Work out the finished part from the listing and answer in its coordinate system (mm). Face numbers are marked on the shaded views. A direction names the side the tool comes from. Coordinates: 2 decimals unless noted, no trailing zeros. Order: outer loops, then holes, each group sorted by start corner. A loop starts at its lowest first (then second) coordinate and runs counter-clockwise, first axis right, second up. Notation, with made-up numbers: M 8.5,10.5 L 35.5,10.5 A10 cw 35.5,27.5 Z; hole C 14,45.5 d4. An arc over 180 degrees is marked long. Use a Markdown table: item, result.
from build123d import *

# Parameters (mm, degrees)
SKETCH1_R           = 15
BOSS_EXTRUDE1_DEPTH = 10
SKETCH2_R           = 7
BOSS_EXTRUDE2_DEPTH = 98
SKETCH4_R           = 15
BOSS_EXTRUDE3_DEPTH = 10


with BuildPart() as part:
    # Sketch1 → Boss-Extrude1 (new body)
    with BuildSketch(Plane(origin=(0, 0, 0), x_dir=(1, 0, 0), z_dir=(0, 1, 0))):
        Circle(SKETCH1_R)
    extrude(amount=-BOSS_EXTRUDE1_DEPTH)

    # Sketch2 → Boss-Extrude2 (add)
    with BuildSketch(Plane.XZ.offset(10)):
        Circle(SKETCH2_R)
    extrude(amount=BOSS_EXTRUDE2_DEPTH)

    # Sketch4 → Boss-Extrude3 (add)
    with BuildSketch(Plane.XZ.offset(108)):
        Circle(SKETCH4_R)
    extrude(amount=-BOSS_EXTRUDE3_DEPTH)


solid = part.part
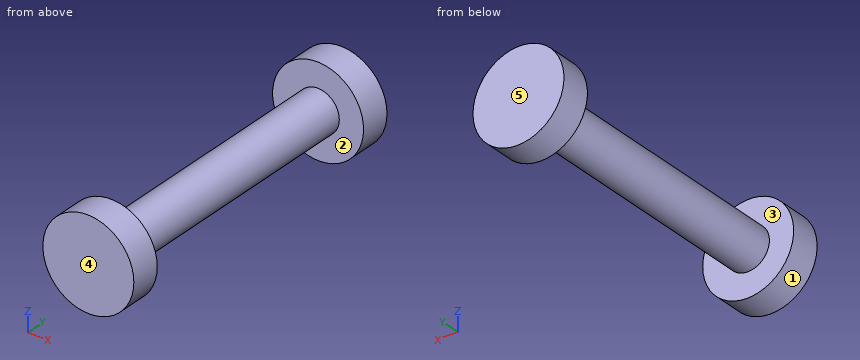
1. Find the intervals of material crossed by probe 1 along Y at (x, z) = (0.5, 11.75); probe 2 along X at (y, z) = (-31, -0.25); probe 3 along Z at (x, y) = (-0.5, -51), in increasing order.
Answers below:
| item | result |
|---|---|
| probe 1 | -108 to -98, -10 to 0 |
| probe 2 | -7 to 7 |
| probe 3 | -6.98 to 6.98 |
2. Section A-A on x = -9 is taken. Determine the outline of the cut face in (y, z), then the cut area to 3 significant figures.
Answers below:
| item | result |
|---|---|
| outline | M -108,-12 L -98,-12 L -98,12 L -108,12 Z; M -10,-12 L 0,-12 L 0,12 L -10,12 Z |
| area | 480 mm² |
3. Flat-ended cylindrical pins translate along their axes: P1, Ø1, axis at x = 5, y = -92, coming from the +Z side; P2, Ø10, axis at y = -76, z = -9.5, coming from the -X side; P3, Ø8, axis at y = -26.5, z = -3, coming from the +X side. Find the tip coordinate at first contact, or state that the pin passes through.
Answers below:
| item | result |
|---|---|
| P1 | z = 5.36 |
| P2 | x = -5.36 |
| P3 | x = 7 |
4. Section D-D on z = 0 is taken. Determine the outline of the cut face in (x, y), then the cut area to 3 significant figures.
Answers below:
| item | result |
|---|---|
| outline | M -15,-108 L 15,-108 L 15,-98 L 7,-98 L 7,-10 L 15,-10 L 15,0 L -15,0 L -15,-10 L -7,-10 L -7,-98 L -15,-98 Z |
| area | 1,830 mm² |
5. Section B-B on z = -8.25 is taken. Determine the outline of the cut face in (x, y), then the cut area to 3 significant figures.
Answers below:
| item | result |
|---|---|
| outline | M -12.53,-108 L 12.53,-108 L 12.53,-98 L -12.53,-98 Z; M -12.53,-10 L 12.53,-10 L 12.53,0 L -12.53,0 Z |
| area | 501 mm² |
6. For a pull along Y with two mould halves and no side action, classify the marked faces 3, 4 and 5 as +Y half, -Y half, draft (parallel to the pull), parting line (faces both ways), or undercut.
Answers below:
| item | result |
|---|---|
| face 3 | undercut |
| face 4 | -Y half |
| face 5 | +Y half |
7. Section C-C on x = 0 is taken. Determine the outline of the cut face in (y, z), then the cut area to 3 significant figures.
Answers below:
| item | result |
|---|---|
| outline | M -108,-15 L -98,-15 L -98,-7 L -10,-7 L -10,-15 L 0,-15 L 0,15 L -10,15 L -10,7 L -98,7 L -98,15 L -108,15 Z |
| area | 1,830 mm² |
8. For the marked faces 1 and 2, determine the directions among +Z, -Z, +X, -X, +Y, -Y from which every point of the face is accessible in a straight line to the end or side of a thin tool.
Answers below:
| item | result |
|---|---|
| face 1 | +Y, -Y |
| face 2 | none |
